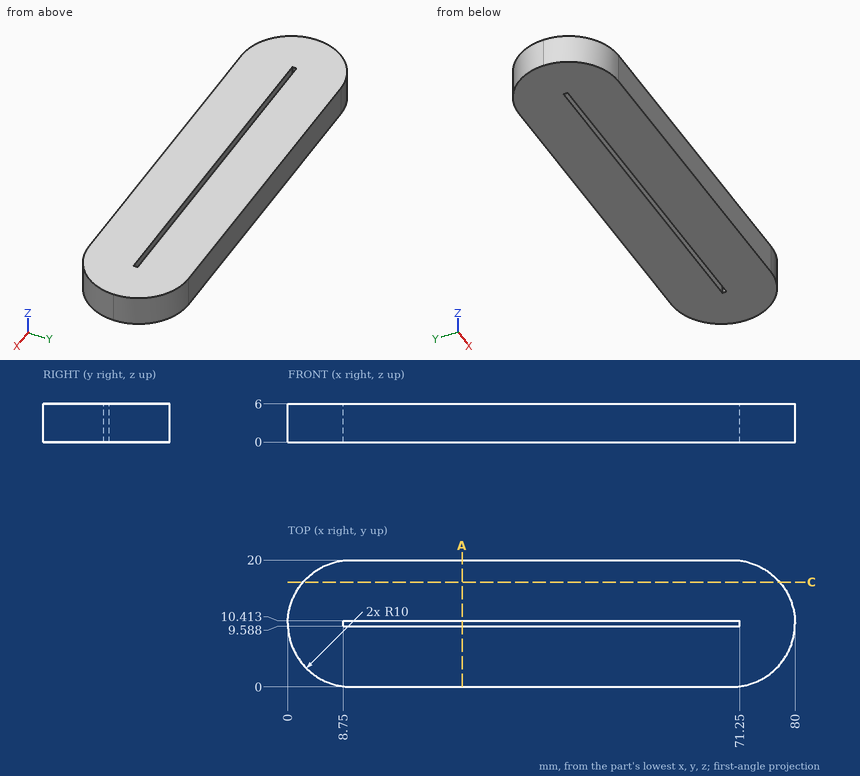
Input: dimensioned drawing with shaded views. Units: mm. Origin: part minimum x, y, z. Round coordinates to 2 decimals unless told otherwise and drop trailing zeros. Loops run counter-clockwise (first coordinate to the right, second up) from the corner with the lowest first, then second, coordinate; pieces in that order, holes last. Notation, with made-up numbers: (4.5, 61.25) -> (16.5, 61.25) arc R22 ccw to (16.5, 68.25) -> close; hole circle Ø10 at (8.5, 9). An arc over 180 degrees is marked (long way). Answer as a JSON object with one key per item and string values. Group by question number.
1) Ray query, L1, parallel to Y at x = 27, z = 2.95; L2, parallel to X at y = 9.75, z = 3.5; L3, parallel to X at y = 10.5, z = 4.65. Return the intervals inside material, ascending.
2) Section query A-A on x = 27.5. Output: boundary loops of the cut face in (y, z).
3) Pin query (flat end, axial travel): pin 1 (1.5 mm diameter, centred on y = 3.5, z = 1, fed in from -X); pin 2 (10 mm diameter, centred on x = 31, y = 6.5, fed in from -Z); pin 3 (1 mm diameter, centred on y = 14, z = 5.5, fed in from +X). Return the tip coordinate at first contact, or that it passes through.
4) Section query C-C on y = 16.5. Output: boundary loops of the cut face in (x, z).
Reply:
{
 "1": {"L1": "y = 0 to 9.59, 10.41 to 20", "L2": "x = 0 to 8.75, 71.25 to 80", "L3": "x = 0.01 to 79.99"},
 "2": {"outline": "(0, 0) -> (9.59, 0) -> (9.59, 6) -> (0, 6) -> close; (10.41, 0) -> (20, 0) -> (20, 6) -> (10.41, 6) -> close"},
 "3": {"pin 1": "stops at x = 1.82", "pin 2": "stops at z = 0", "pin 3": "stops at x = 79.37"},
 "4": {"outline": "(2.4, 0) -> (77.6, 0) -> (77.6, 6) -> (2.4, 6) -> close"}
}
